Geometry: final body of the model. Coordinates: model frame, mm. Face numbers are marked on the shaded views. A direction names the side the tool comes from. Coordinates: 2 decimals unless noted, no trailing zeros. Order: outer loops, then holes, each group sorted by start corner. A loop starts at its lowest first (then second) coordinate and runs counter-clockwise, first axis right, second up. Notation, with made-up numbers: M -5.75,49.5 L 24.25,49.5 A13 ccw 24.25,54.5 Z; hole C -14.75,61.25 d9. An arc over 180 degrees is marked long. Use CSV: the item, a comma, the result in double quotes. Start each with the question number.
Q1. Section query A-A, the plane z = 6.75. Output: boundary loops of the cut face in (x, y), and give its area (3 significant figures).
Q2. First-contact query: P1, Ø0.6, axis at x = 0, z = 0.5, coming from the +Y side; P2, Ø2, axis at y = 1.5, z = 7.5, coming from the +X side; P3, Ø1.5, axis at x = -1.5, z = 6, coming from the -Y side. Flat tips, straight axial feed; report the tip coordinate or a pass-through.
Q3. Access query for the marked faces 1, 2 and 3. Directions: +Z, -Z, +X, -X, +Y, -Y. A direction counts if a zero-diameter tool reaches every point of the face in a straight line with its end or side. Return the directions, or none.
Q4. Ray query, probe 1 along X at (y, z) = (0.1, 13.5); probe 2 along X at (y, z) = (-0.55, 13.25); probe 3 along Y at (x, z) = (-0.45, 10). Return the intervals inside material, ascending.
from build123d import *

# Parameters (mm, degrees)
F1_R     = 2.75
F1_R_2   = 1.5
F2_DEPTH = 2
F3_START = 1.5
F3_DEPTH = 0.5
F4_START = 2
F4_DEPTH = 13
F5_SIZE2 = 1.25
F5_SIZE  = 1.25
F6_R     = 0.25


# Not quite as in the source:
# - a feature names something its author has since deleted; it is built from what else it names


with BuildPart() as f2:
    # F1 (on Top) → F2 (new body)
    with BuildSketch(Plane.XY):
        Circle(F1_R)
        Circle(F1_R_2, mode=Mode.SUBTRACT)
        Circle(F1_R_2)
        Polygon((-0.5773502692, -1), (-1.1547005384, 0), (-0.5773502692, 1), (0.5773502692, 1), (1.1547005384, 0), (0.5773502692, -1), align=None, mode=Mode.SUBTRACT)
    extrude(amount=F2_DEPTH)

    # F1 (on Top) → F3 (join)
    with BuildSketch(Plane.XY.offset(F3_START)):
        Polygon((-0.5773502692, 1), (-1.1547005384, 0), (-0.5773502692, -1), (0.5773502692, -1), (1.1547005384, 0), (0.5773502692, 1), align=None)
    extrude(amount=F3_DEPTH)

    # F1 (on Top) → F4 (join)
    with BuildSketch(Plane.XY.offset(F4_START)):
        Circle(F1_R_2)
        Polygon((-0.5773502692, -1), (-1.1547005384, 0), (-0.5773502692, 1), (0.5773502692, 1), (1.1547005384, 0), (0.5773502692, -1), align=None, mode=Mode.SUBTRACT)
        Polygon((-0.5773502692, 1), (-1.1547005384, 0), (-0.5773502692, -1), (0.5773502692, -1), (1.1547005384, 0), (0.5773502692, 1), align=None)
    extrude(amount=F4_DEPTH)

    # F5
    f5_edges = [f2.edges().sort_by_distance(p)[0] for p in [
        (-2.75, 0, 0),
    ]]
    chamfer(f5_edges, length=F5_SIZE, length2=F5_SIZE2)

    # F6
    f6_edges = [f2.edges().sort_by_distance(p)[0] for p in [
        (-2.75, 0, 2),
        (-1.5, 0, 2),
        (-1.5, 0, 0),
        (-2.75, 0, 1.25),
    ]]
    fillet(f6_edges, radius=F6_R)


solid = f2.part
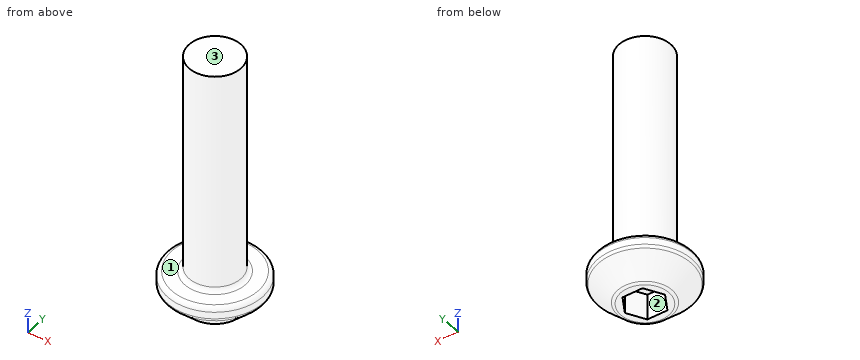
Responses:
1,outline,"C 0,0 d3"
1,area,"7.07 mm²"
2,P1,"stops at y = 2.3"
2,P2,"stops at x = 1.41"
2,P3,"stops at y = -1.3"
3,face 1,"+Z"
3,face 2,"-Z"
3,face 3,"+Z, +X, -X, +Y, -Y"
4,probe 1,"x = -1.5 to 1.5"
4,probe 2,"x = -1.4 to 1.4"
4,probe 3,"y = -1.43 to 1.43"
